```python
from build123d import *

# Parameters (mm, degrees)
F0_R     = 50
F0_R_2   = 45
F0_R_3   = 40
F0_R_4   = 35
F1_DEPTH = 90
F2_DEPTH = 100
F3_DEPTH = 10


with BuildPart() as f1:
    # F0 (on Top) → F1 (new body)
    with BuildSketch(Plane.XY):
        with Locations((-87.7033099532, -2.8714591172)):
            Circle(F0_R)
        with Locations((-87.7033099532, -2.8714591172)):
            Circle(F0_R_2, mode=Mode.SUBTRACT)
        with Locations((-87.7033099532, -2.8714591172)):
            Circle(F0_R_2)
        with Locations((-87.7033099532, -2.8714591172)):
            Circle(F0_R_3, mode=Mode.SUBTRACT)
        with Locations((-87.7033099532, -2.8714591172)):
            Circle(F0_R_3)
        with Locations((-87.7033099532, -2.8714591172)):
            Circle(F0_R_4, mode=Mode.SUBTRACT)
    extrude(amount=F1_DEPTH)

    # F0 (on Top) → F2 (join)
    with BuildSketch(Plane.XY):
        with Locations((-87.7033099532, -2.8714591172)):
            Circle(F0_R_2)
        with Locations((-87.7033099532, -2.8714591172)):
            Circle(F0_R_3, mode=Mode.SUBTRACT)
    extrude(amount=F2_DEPTH)

    # F0 (on Top) → F3 (cut)
    with BuildSketch(Plane.XY):
        with Locations((-87.7033099532, -2.8714591172)):
            Circle(F0_R_2)
        with Locations((-87.7033099532, -2.8714591172)):
            Circle(F0_R_3, mode=Mode.SUBTRACT)
    extrude(amount=F3_DEPTH, mode=Mode.SUBTRACT)


solid = f1.part
```
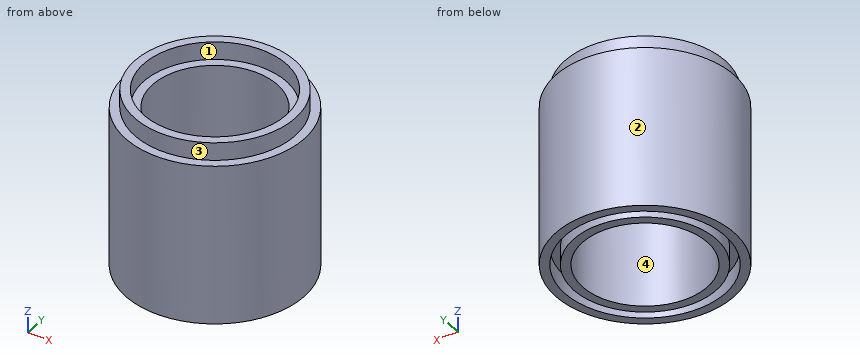
Build history of the part. All positions in model axes, mm. Face numbers are marked on the shaded views. A direction names the side the tool comes from. Give positions to 0.01 mm unless a question says otherwise; leave off trailing zeros. Loops run counter-clockwise (first coordinate to the right, second up) from the corner with the lowest first, then second, coordinate; pieces in that order, holes last.
Item 1: Flat gauge pins, fed straight in: pin 1 (2 mm diameter, centred on x = -89, z = 21.5, fed in from -Y); pin 2 (5 mm diameter, centred on x = -98, z = 36.5, fed in from -Y); pin 3 (2 mm diameter, centred on y = 37, z = 24, fed in from -X). Where does each tip first touch, or does it go through?
Answers follow:
pin 1: stops at y = -52.87
pin 2: stops at y = -52.26
pin 3: stops at x = -119.15
Item 2: Drill centre lines: line 1 (Y direction, x = -85, z = 4.5); line 2 (X direction, y = 9, z = 61); line 3 (Z direction, x = -50, y = 0.5). Where is each one in solid material? Low to high.
Answers follow:
line 1: y = -52.8 to -47.79, -42.78 to -37.77, 32.02 to 37.04, 42.05 to 47.06
line 2: x = -136.27 to -120.63, -54.78 to -39.13
line 3: z = 0 to 90
Item 3: Slice it at B-B, the plane y = 21.5. List the corners of the cut face in (x, z), and give its area (3 significant figures).
Answers follow:
outline: (-131.36, 0) - (-125.53, 0) - (-125.53, 10) - (-119.42, 10) - (-119.42, 0) - (-112.82, 0) - (-112.82, 90) - (-119.42, 90) - (-119.42, 100) - (-125.53, 100) - (-125.53, 90) - (-131.36, 90) - close; (-62.58, 0) - (-55.99, 0) - (-55.99, 10) - (-49.87, 10) - (-49.87, 0) - (-44.05, 0) - (-44.05, 90) - (-49.87, 90) - (-49.87, 100) - (-55.99, 100) - (-55.99, 90) - (-62.58, 90) - close
area: 3,340 mm2
Item 4: Which spindle directions (+Z, -Z, +X, -X, +Y, -Y) get a long thin tool onto all of the face, cutting with end or side? Do the marked faces 3 and 4. Say none if no direction does.
Answers follow:
face 3: +Z
face 4: +Z, -Z
Item 5: Slice it at C-C, the plane z = 84.5. List the corners of the cut face in (x, y), and give its area (3 significant figures).
Answers follow:
outline: circle Ø100 at (-87.7, -2.87); hole circle Ø70 at (-87.7, -2.87)
area: 4,010 mm2
Item 6: Pull direction Y, two halves, no side cores. Call the marked faces 1 and 2: released by +Y, released by -Y, zero draft, split by the parting line, or undercut.
Answers follow:
face 1: undercut
face 2: split by the parting line
Item 7: Slice it at A-A, the plane x = -115.5. List the corners of the cut face in (y, z), and give its area (3 significant figures).
Answers follow:
outline: (-44.43, 0) - (-38.26, 0) - (-38.26, 10) - (-31.64, 10) - (-31.64, 0) - (-24.14, 0) - (-24.14, 90) - (-31.64, 90) - (-31.64, 100) - (-38.26, 100) - (-38.26, 90) - (-44.43, 90) - close; (18.4, 0) - (25.89, 0) - (25.89, 10) - (32.52, 10) - (32.52, 0) - (38.69, 0) - (38.69, 90) - (32.52, 90) - (32.52, 100) - (25.89, 100) - (25.89, 90) - (18.4, 90) - close
area: 3,650 mm2
